from build123d import *

# Parameters (mm, degrees)
BOSS_EXTRUDE2_DEPTH = 331.382
SKETCH3_W           = 66
SKETCH3_H           = 122
CUT_EXTRUDE2_DEPTH  = 128.0000001
SKETCH4_W           = 80
SKETCH4_H           = 10
CUT_EXTRUDE3_DEPTH  = 332.3820001
SKETCH5_W           = 260
SKETCH5_H           = 70
CUT_EXTRUDE4_DEPTH  = 332.3820001


with BuildPart() as part:
    # Sketch2 → Boss-Extrude2 (new body)
    with BuildSketch(Plane.XY):
        with BuildLine():
            Line((-127, 127), (127, 127))
            add(Edge.make_bspline(
                [(-127, 127), (0, -127), (127, 127)],
                knots=[0.056028396, 0.056028396, 0.056028396, 0.943971604, 0.943971604, 0.943971604], degree=2))
        make_face()
    extrude(amount=BOSS_EXTRUDE2_DEPTH)

    # Sketch3 → Cut-Extrude2 (cut, through all)
    with BuildSketch(Plane(origin=(0, 127, 0), x_dir=(1, 0, 0), z_dir=(0, 1, 0))):
        with Locations((0, -82.8455)):
            Rectangle(SKETCH3_W, SKETCH3_H)
        with Locations((0, -248.5365)):
            Rectangle(SKETCH3_W, SKETCH3_H)
    extrude(amount=-CUT_EXTRUDE2_DEPTH, mode=Mode.SUBTRACT)

    # Sketch4 → Cut-Extrude3 (cut, through all)
    with BuildSketch(Plane(origin=(0, 0, 0), x_dir=(-1, 0, 0), z_dir=(0, 0, -1))):
        with Locations((0, 5)):
            Rectangle(SKETCH4_W, SKETCH4_H)
    extrude(amount=-CUT_EXTRUDE3_DEPTH, mode=Mode.SUBTRACT)

    # Sketch5 → Cut-Extrude4 (cut, through all)
    with BuildSketch(Plane.XY.offset(331.382)):
        with Locations((0, 95.8)):
            Rectangle(SKETCH5_W, SKETCH5_H)
    extrude(amount=-CUT_EXTRUDE4_DEPTH, mode=Mode.SUBTRACT)


solid = part.part
CAD build for the part. Positions are in the model's coordinates, mm. A direction names the side the tool comes from. Coordinates: 2 decimals unless noted, no trailing zeros. Write each loop counter-clockwise with the first axis right and the second up, starting at its lowest first coordinate (ties: lowest second). Pieces come first, ordered by that corner, then holes. Notation, with made-up numbers: M 35.5,35 L 67.5,35 A18 ccw 67.5,39 Z; hole C 31.25,74.5 d4. An arc over 180 degrees is marked long. Return JSON: item names as keys, results as strings.
Item 1: Probe line 1 (Z direction, x = 2, y = 58); line 2 (X direction, y = 31, z = 246); line 3 (X direction, y = 58, z = 72). List the from-to ranges inside material, lowest first. Write a range as from..to.
Findings below:
{"line 1": "z = 0..21.85, 143.85..187.54, 309.54..331.38", "line 2": "x = -62.75..-33, 33..62.75", "line 3": "x = -85.83..-33, 33..85.83"}
Item 2: Slice it at B-B, the plane y = 50. State how many separate pieces and enclosed holes the cut face has, and give its area (3 significant figures).
Findings below:
{"separate pieces": "1", "enclosed holes": "2", "area": "36,700 mm2"}
Item 3: Slice it at A-A, the plane x = -8.5. Write the cut outline in (y, z), and give its area (3 significant figures).
Findings below:
{"outline": "M 10,0 L 60.8,0 L 60.8,21.85 L 10,21.85 Z; M 10,143.85 L 60.8,143.85 L 60.8,187.54 L 10,187.54 Z; M 10,309.54 L 60.8,309.54 L 60.8,331.38 L 10,331.38 Z", "area": "4,440 mm2"}
Item 4: Which spindle directions (+Z, -Z, +X, -X, +Y, -Y) get a long thin tool onto all of the face, cutting with end or side? Do faces 3 (the flat face through (1, 41, 0)), 4 (the flat face through (0, 36, 187.536)). Say none if no direction does.
Findings below:
{"face 3": "-Z, +X, -X, +Y, -Y", "face 4": "+Y, -Y"}
Item 5: Two-plate mould, pull along X, no slides. Class faces 1 (the flat face through (33, 36, 249)), 2 (the flat face through (-1, 60.8, 168)): +X half, -X half, draft (parallel to the pull), parting line (faces both ways), or undercut.
Findings below:
{"face 1": "undercut", "face 2": "draft"}
Item 6: Drop flat-ended pins along their axis: pin 1 Ø3 at (y, z) = (16.5, 105.5) entering from -X; pin 2 Ø4 at (y, z) = (18, 245.5) entering from +X. Give the stop position or say it passes through.
Findings below:
{"pin 1": "stops at x = -47.81", "pin 2": "stops at x = 50.4"}
